For this review, take the finished solid that the model builds, in its own axes (mm). Round coordinates to 2 decimals unless told otherwise and drop trailing zeros. Use one line per item in the form item = value. Start each with the question number.
Item 1: Draft analysis for pull direction X (two halves, no side actions). For faces 1 (the flat face through (10, 200, -1)), 2 (the cylindrical face through (-15.02, 198.5, 47.69)), 3 (the cylindrical face through (4.214, 180.509, -0.553)), state which applies: released by +X, released by -X, zero draft, split by the parting line, or undercut.
Item 2: For line 1 (Z direction, x = -32, y = 129); line 2 (X direction, y = 178, z = 0); line 3 (X direction, y = 185.5, z = 0), list the stretches that pass through material, from the lowest coordinate up. Write a range as [from, to].
Item 3: For P1, Ø2, axis at y = 178, z = -14.5, coming from the -X side; P2, Ø1, axis at y = 66.5, z = -54.5, coming from the -X side; P3, Ø7, axis at x = 0, z = 0, coming from the -Y side; P4, Ø1, axis at x = 23.5, y = 69, coming from the +Z side, all flat-tipped, find the tip position at first contact; note any pin that passes through.
from build123d import *

# Parameters (mm, degrees)
SKETCH6_R          = 4.25
CUT_EXTRUDE1_DEPTH = 237.394879975


with BuildPart() as part:
    # Sketch2 → Revolve1 (revolve)
    with BuildSketch(Plane(origin=(0, 0, 0), x_dir=(0, 0, -1), z_dir=(1, 0, 0))):
        with BuildLine():
            Line((-47, 200), (-47, 196.952633809))
            ThreePointArc((-47, 196.952633809), (-45.020836212, 183.457289916), (-39.250029499, 171.098520319))
            ThreePointArc((-39.250029499, 171.098520319), (-32.165314943, 148.143950557), (-38.499883067, 124.971149691))
            add(Edge.make_bspline(
                [(-38.499883067, 124.971149691), (-39.004530717, 124.147950453), (-39.989837427, 122.509882381), (-41.987103434, 119.066741734), (-44.476625137, 114.542174666), (-47.469272443, 108.73134572), (-51.458823728, 100.486184281), (-56.445386005, 89.243791761), (-62.422969316, 74.260784727), (-68.39139954, 57.78817126), (-73.355476081, 42.822187789), (-77.320473203, 30.10613441), (-80.290300516, 20.200019419), (-82.763970951, 11.629508828), (-84.647070901, 4.923001543), (-85.564233648, 1.602436154), (-85.985445094, 0.065829354), (-86.003484285, -2.71e-07)],
                knots=[0.502863577, 0.502863577, 0.502863577, 0.502863577, 0.502970965, 0.503078353, 0.503293128, 0.503507904, 0.50372268, 0.504152231, 0.504581782, 0.505011333, 0.505440885, 0.50565566, 0.505870436, 0.506085211, 0.506192599, 0.506280364, 0.506284289, 0.506284289, 0.506284289, 0.506284289], degree=3))
            Line((-86.003484285, -2.71e-07), (-89.113801103, 0))
            add(Edge.make_bspline(
                [(-41.057539829, 126.539075674), (-65.366339288, 86.885695354), (-89.113801103, 0)],
                knots=[0, 0, 0, 1, 1, 1], degree=2))
            ThreePointArc((-41.057539829, 126.539075674), (-35.16491832, 148.095169564), (-41.755350531, 169.448257756))
            ThreePointArc((-41.755350531, 169.448257756), (-47.894506608, 182.595884987), (-50, 196.952633809))
            Line((-50, 196.952633809), (-50, 200))
            Line((-50, 200), (-47, 200))
        make_face()
    revolve(axis=Axis((0, 180, 0), (0, -1, 0)))

    # Sketch5 → Revolve2 (revolve)
    with BuildSketch(Plane(origin=(0, 0, 0), x_dir=(0, 0, -1), z_dir=(1, 0, 0)), mode=Mode.PRIVATE) as revolve2_sk:
        with BuildLine():
            Line((-33.861088957, 130.854414053), (-3, 161.71550301))
            Line((-3, 161.71550301), (0, 161.71550301))
            Line((0, 161.71550301), (0, 200))
            Line((0, 200), (-47, 200))
            Line((-47, 200), (-47, 196.952633809))
            ThreePointArc((-47, 196.952633809), (-45.020836212, 183.457289916), (-39.250029499, 171.098520319))
            ThreePointArc((-39.250029499, 171.098520319), (-32.165314943, 148.143950557), (-38.499883067, 124.971149691))
            ThreePointArc((-38.499883067, 124.971149691), (-36.353838994, 128.049465988), (-33.861088957, 130.854414053))
        make_face()
    revolve(revolve2_sk.sketch.rotate(Axis((0, -1000, 0), (0, 1, 0)), 180), axis=Axis((0, -1000, 0), (0, 1, 0)))

    # Sketch6 → Cut-Extrude1 (cut, through all)
    with BuildSketch(Plane(origin=(0, 200, 0), x_dir=(1, 0, 0), z_dir=(0, 1, 0))):
        with Locations(Location((0, 0, 0), (0, 0, 270))):
            Circle(SKETCH6_R)
    extrude(amount=-CUT_EXTRUDE1_DEPTH, mode=Mode.SUBTRACT)


solid = part.part
Calculated:
q1.face_1 = zero draft
q1.face_2 = split by the parting line
q1.face_3 = undercut
q2.line_1 = [-23.44, -15.54], [15.54, 23.44]
q2.line_2 = [-46.27, -4.25], [4.25, 46.27]
q2.line_3 = [-48.67, -4.25], [4.25, 48.67]
q3.P1 = -44.47
q3.P2 = -42.05
q3.P3 = through
q3.P4 = 63.54
